Part print with two shaded views. Sizes in mm from the minimum x, y, z corner. Give positions to 0.01 mm unless a question says otherwise; leave off trailing zeros. Write each loop counter-clockwise with the first axis right and the second up, starting at its lowest first coordinate (ties: lowest second). Pieces come first, ordered by that corner, then holes. Notation, with made-up numbers: (83.25, 51.25) - (141.25, 51.25) arc R19 cw to (141.25, 75.25) - close; hole circle Ø4 at (10.25, 14.25). An arc over 180 degrees is marked (long way). One line per item, written item: value. Start each with the question number.
(1) Mould opens along Z. For the marked faces 1 and 2 say: pulls with the +Z half, pulls with the -Z half, needs draft (parallel to the pull), parting line crosses it, or undercut.
(2) Cut at B-B, the plane x = 18. State how many separate pieces and enclosed holes the cut face has, and give its area (3 significant figures).
(3) Probe L1, parallel to X at y = 227.5, z = 2.75; L2, parallel to X at y = 211.5, z = 1.5 (1 decimal); L3, parallel to Y at x = 127.5, z = 0.75. List the from-to ranges inside material, lowest first.
(4) Cut at A-A, the plane y = 270.5. List the corners of the cut face in (x, z).
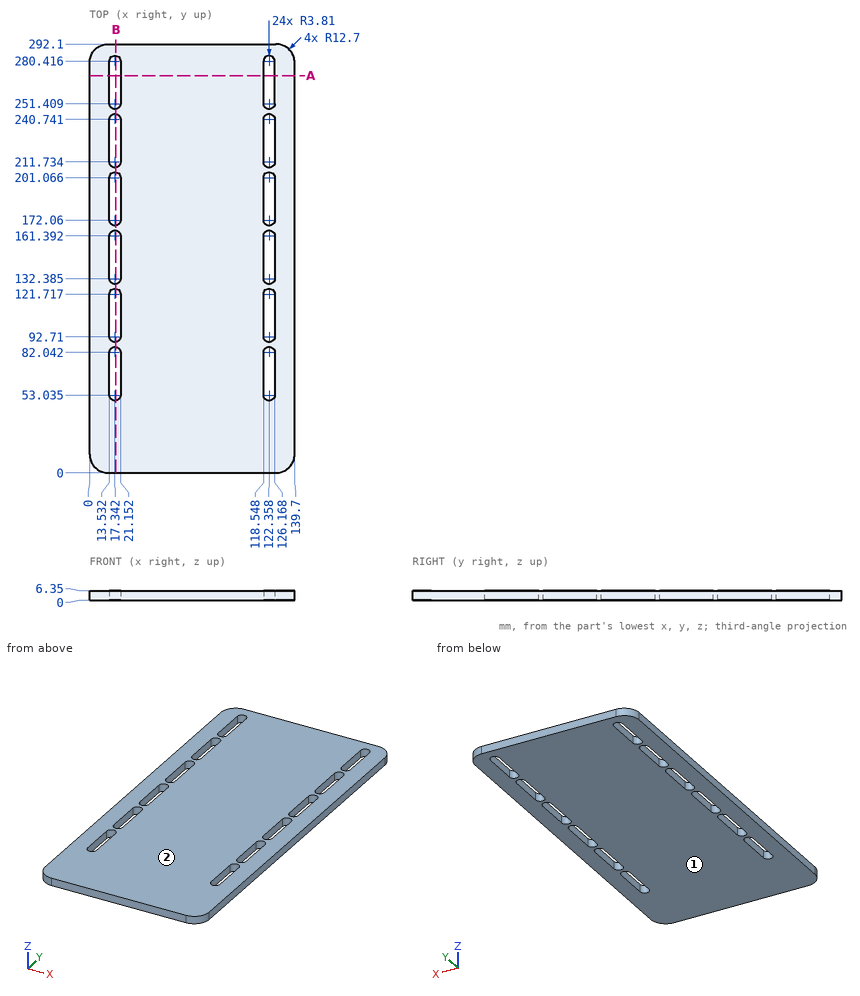
Answers follow:
1. face 1: pulls with the -Z half
1. face 2: pulls with the +Z half
2. separate pieces: 7
2. enclosed holes: 0
2. area: 464 mm²
3. L1: x = 0 to 13.53, 21.15 to 118.55, 126.17 to 139.7
3. L2: x = 0 to 13.5, 21.1 to 118.6, 126.2 to 139.7
3. L3: y = 0.01 to 292.09
4. outline: (0, 0) - (13.53, 0) - (13.53, 6.35) - (0, 6.35) - close; (21.15, 0) - (118.55, 0) - (118.55, 6.35) - (21.15, 6.35) - close; (126.17, 0) - (139.7, 0) - (139.7, 6.35) - (126.17, 6.35) - close
